Geometry: final body of the model. Coordinates: model frame, mm. Coordinates: 2 decimals unless noted, no trailing zeros. Order: outer loops, then holes, each group sorted by start corner. A loop starts at its lowest first (then second) coordinate and runs counter-clockwise, first axis right, second up. Notation, with made-up numbers: (-37, -2) - (17, -2) arc R31 ccw to (17, 31) - close; hole circle Ø9 at (-7, -7.5). An arc over 180 degrees is marked (long way). Use a Markdown table: item, result. Add a question column.
```python
from build123d import *

# Parameters (mm, degrees)
BOSS_EXTRUDE1_DEPTH         = 3.175
F_1_2_CLEARANCE_SLOT1_DEPTH = 3.175
F_3_8_CLEARANCE_HOLE1_D     = 10.0838


# Read off the part's stored shape, not the designer's step: 1/2 Clearance Slot1
with BuildPart() as part:
    # Sketch1 → Boss-Extrude1 (new body)
    with BuildSketch(Plane(origin=(0, 0, 0), x_dir=(1, 0, 0), z_dir=(0, 1, 0))):
        with BuildLine():
            Line((76.2, 0), (330.2, 0))
            ThreePointArc((330.2, 0), (384.081536726, 22.318463274), (406.4, 76.2))
            Line((406.4, 76.2), (406.4, 228.6))
            ThreePointArc((406.4, 228.6), (384.081536726, 282.481536726), (330.2, 304.8))
            Line((330.2, 304.8), (76.2, 304.8))
            ThreePointArc((76.2, 304.8), (22.318463274, 282.481536726), (0, 228.6))
            Line((0, 228.6), (0, 76.2))
            ThreePointArc((0, 76.2), (22.318463274, 22.318463274), (76.2, 0))
        make_face()
    extrude(amount=BOSS_EXTRUDE1_DEPTH)

    # 1/2 Clearance Slot1 outline → 1/2 Clearance Slot1 (cut)
    with BuildSketch(Plane(origin=(0, 0, 0), x_dir=(1, 0, 0), z_dir=(0, 1, 0))):
        with BuildLine():
            Line((336.94624, 145.65376), (350.44126, 145.65376))
            ThreePointArc((350.44126, 145.65376), (357.1875, 152.4), (350.44126, 159.14624))
            Line((350.44126, 159.14624), (336.94624, 159.14624))
            ThreePointArc((336.94624, 159.14624), (330.2, 152.4), (336.94624, 145.65376))
        make_face()
        with BuildLine():
            ThreePointArc((69.45376, 145.65376), (76.2, 152.4), (69.45376, 159.14624))
            Line((69.45376, 159.14624), (55.95874, 159.14624))
            ThreePointArc((55.95874, 159.14624), (49.2125, 152.4), (55.95874, 145.65376))
            Line((55.95874, 145.65376), (69.45376, 145.65376))
        make_face()
    extrude(amount=F_1_2_CLEARANCE_SLOT1_DEPTH, mode=Mode.SUBTRACT)

    # 3/8 Clearance Hole1 (through all)
    with Locations(Plane(origin=(0, 3.175, 0), x_dir=(1, 0, 0), z_dir=(0, 1, 0))):
        with Locations((138.90625, 88.9), (267.49375, 215.9), (267.49375, 88.9), (138.90625, 215.9)):
            Hole(F_3_8_CLEARANCE_HOLE1_D / 2)


solid = part.part
```
1) Section A-A (y = 1). Return loops of the section in (x, z).
2) Ray query, line 1 along X through (y, z) = (1.7, -88.9); line 2 along X through (y, z) = (2.15, -218.5); line 3 along X through (y, z) = (0.8, -232). Return the intervals inside material, ascending.
3) Draft query along X for faces 1 (the face through (384.671, 1.565, -281.886)), 2 (the face through (272.53, 1.57, -216.12)), 3 (the face through (21.729, 1.565, -22.914)), 4 (the face through (200, 3.175, -155)). Return one class per face: pulls with the +X half, pulls with the -X half, needs draft (parallel to the pull), parting line crosses it, or undercut.
4) Section B-B (z = -215.9). Return loops of the section in (x, y) (3 decimals).
5) Pin query (flat end, axial travel): pin 1 (1.6 mm diameter, centred on x = 346, y = 1.5, fed in from -Z); pin 2 (1.6 mm diameter, centred on x = 62, y = 2, fed in from +Z). Return the tip coordinate at first contact, or that it passes through.
6) Section D-D (z = -42.5). Return loops of the section in (x, y) (3 decimals), then the cut area to 3 significant figures.
7) Section C-C (z = -152.4). Return loops of the section in (x, y) (1 decimal), then the cut area to 3 significant figures.
Values follow:
| question | item | result |
|---|---|---|
| 1 | outline | (0, -228.6) arc R76.2 ccw to (76.2, -304.8) - (330.2, -304.8) arc R76.2 ccw to (406.4, -228.6) - (406.4, -76.2) arc R76.2 ccw to (330.2, 0) - (76.2, 0) arc R76.2 ccw to (0, -76.2) - close; hole (55.96, -159.15) - (69.45, -159.15) arc R6.75 ccw to (69.45, -145.65) - (55.96, -145.65) arc R6.75 ccw to start; hole circle Ø10.08 at (138.91, -215.9); hole circle Ø10.08 at (138.91, -88.9); hole circle Ø10.08 at (267.49, -215.9); hole circle Ø10.08 at (267.49, -88.9); hole (336.95, -159.15) - (350.44, -159.15) arc R6.75 ccw to (350.44, -145.65) - (336.95, -145.65) arc R6.75 ccw to start |
| 2 | line 1 | x = 0 to 133.86, 143.95 to 262.45, 272.54 to 406.4 |
| 2 | line 2 | x = 0 to 134.59, 143.23 to 263.17, 271.81 to 406.4 |
| 2 | line 3 | x = 0.08 to 406.32 |
| 3 | face 1 | pulls with the +X half |
| 3 | face 2 | undercut |
| 3 | face 3 | pulls with the -X half |
| 3 | face 4 | needs draft |
| 4 | outline | (0, 0) - (133.864, 0) - (133.864, 3.175) - (0, 3.175) - close; (143.948, 0) - (262.452, 0) - (262.452, 3.175) - (143.948, 3.175) - close; (272.536, 0) - (406.4, 0) - (406.4, 3.175) - (272.536, 3.175) - close |
| 5 | pin 1 | stops at z = -303.31 |
| 5 | pin 2 | stops at z = -1.19 |
| 6 | outline | (7.857, 0) - (398.543, 0) - (398.543, 3.175) - (7.857, 3.175) - close |
| 6 | area | 1,240 mm² |
| 7 | outline | (0, 0) - (49.2, 0) - (49.2, 3.2) - (0, 3.2) - close; (76.2, 0) - (330.2, 0) - (330.2, 3.2) - (76.2, 3.2) - close; (357.2, 0) - (406.4, 0) - (406.4, 3.2) - (357.2, 3.2) - close |
| 7 | area | 1,120 mm² |
